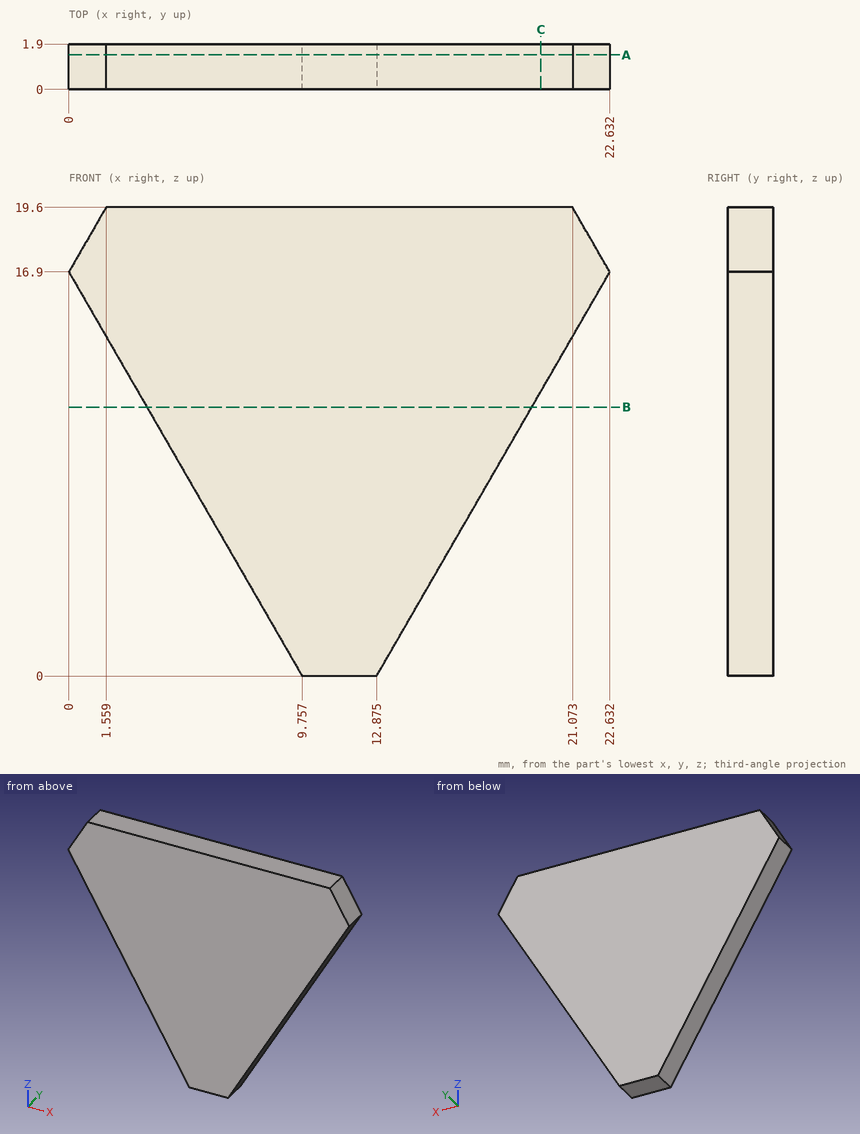
Could you check a few things on this drawing? It's one solid part, dimensions in mm from its lowest x, y, z. Round coordinates to 2 decimals unless told otherwise and drop trailing zeros. Loops run counter-clockwise (first coordinate to the right, second up) from the corner with the lowest first, then second, coordinate; pieces in that order, holes last.
Q1. For P1, Ø1, axis at x = 13.5, y = 1.5, coming from the -Z side (1 decimal); P2, Ø1, axis at x = 14.5, y = 1, coming from the -Z side, each with a flat end and sliding along its axis, tell me the tip position at first contact or that it passes through.
Q2. Please list where these lines run through material, in increasing order: L1, parallel to X at y = 0.85, z = 3.75; L2, parallel to X at y = 1.4, z = 1; L3, parallel to Z at x = 21.5, y = 1.6.
Q3. I want a section at B-B (z = 11.25). Write out the boundary of the cut face in (x, y), and give its area (3 significant figures).
Q4. I want a section at A-A (y = 1.45). Write out the boundary of the cut face in (x, z) (1 decimal).
Q5. I want a section at C-C (x = 19.75). Write out the boundary of the cut face in (y, z), and give its area (3 significant figures).
Answer below:
1. P1: stops at z = 0.2
1. P2: stops at z = 1.95
2. L1: x = 7.59 to 15.04
2. L2: x = 9.18 to 13.45
2. L3: z = 14.94 to 18.86
3. outline: (3.26, 0) - (19.37, 0) - (19.37, 1.9) - (3.26, 1.9) - close
3. area: 30.6 mm2
4. outline: (0, 16.9) - (9.8, 0) - (12.9, 0) - (22.6, 16.9) - (21.1, 19.6) - (1.6, 19.6) - close
5. outline: (0, 11.91) - (1.9, 11.91) - (1.9, 19.6) - (0, 19.6) - close
5. area: 14.6 mm2
